Could you check a few things on this model? Use its own coordinates, in mm. Round coordinates to 2 decimals unless told otherwise and drop trailing zeros. Order: outer loops, then holes, each group sorted by start corner. A loop starts at its lowest first (then second) coordinate and runs counter-clockwise, first axis right, second up. Notation, with made-up numbers: (-15.5, 14) - (7.5, 14) arc R7 ccw to (7.5, 18) - close; hole circle Ø4 at (-1.5, 52.25). An arc over 180 degrees is marked (long way). Use one line per item in the form item = value.
from build123d import *

# Parameters (mm, degrees)
ESQUISSE1_W             = 366
ESQUISSE1_H             = 166
ESQUISSE1_R             = 2.2
ESQUISSE1_R_2           = 4.5
ESQUISSE1_R_3           = 6.5
BOSS_EXTRU_1_DEPTH      = 3
ESQUISSE2_OUTSIDE_W     = 448.38
ESQUISSE2_OUTSIDE_H     = 248.38
ESQUISSE2_OUTSIDE_W_2   = 222
ESQUISSE2_OUTSIDE_H_2   = 48
ENL_V_MAT_EXTRU_1_DEPTH = 4
CONG_1_R                = 6


with BuildPart() as part:
    # Esquisse1 → Boss.-Extru.1 (new body)
    with BuildSketch(Plane.XY):
        with Locations((183, 83)):
            Rectangle(ESQUISSE1_W, ESQUISSE1_H)
        with Locations((13, 153)):
            Circle(ESQUISSE1_R, mode=Mode.SUBTRACT)
        with Locations((13, 13)):
            Circle(ESQUISSE1_R, mode=Mode.SUBTRACT)
        with Locations((13, 83)):
            Circle(ESQUISSE1_R, mode=Mode.SUBTRACT)
        with Locations((173, 153)):
            Circle(ESQUISSE1_R, mode=Mode.SUBTRACT)
        with Locations((193, 83)):
            Circle(ESQUISSE1_R, mode=Mode.SUBTRACT)
        with Locations((173, 83)):
            Circle(ESQUISSE1_R, mode=Mode.SUBTRACT)
        with Locations((193, 153)):
            Circle(ESQUISSE1_R, mode=Mode.SUBTRACT)
        with Locations((353, 83)):
            Circle(ESQUISSE1_R, mode=Mode.SUBTRACT)
        with Locations((353, 13)):
            Circle(ESQUISSE1_R, mode=Mode.SUBTRACT)
        with Locations((353, 153)):
            Circle(ESQUISSE1_R, mode=Mode.SUBTRACT)
        with Locations((193, 13)):
            Circle(ESQUISSE1_R, mode=Mode.SUBTRACT)
        with Locations((173, 13)):
            Circle(ESQUISSE1_R, mode=Mode.SUBTRACT)
        with Locations((270.5, 83)):
            Circle(ESQUISSE1_R_2, mode=Mode.SUBTRACT)
        with Locations((95.5, 83)):
            Circle(ESQUISSE1_R_2, mode=Mode.SUBTRACT)
        with Locations((77.5, 101)):
            Circle(ESQUISSE1_R, mode=Mode.SUBTRACT)
        with Locations((113.5, 101)):
            Circle(ESQUISSE1_R, mode=Mode.SUBTRACT)
        with Locations((77.5, 65)):
            Circle(ESQUISSE1_R, mode=Mode.SUBTRACT)
        with Locations((113.5, 65)):
            Circle(ESQUISSE1_R, mode=Mode.SUBTRACT)
        with Locations((288.5, 65)):
            Circle(ESQUISSE1_R, mode=Mode.SUBTRACT)
        with Locations((252.5, 65)):
            Circle(ESQUISSE1_R, mode=Mode.SUBTRACT)
        with Locations((252.5, 101)):
            Circle(ESQUISSE1_R, mode=Mode.SUBTRACT)
        with Locations((288.5, 101)):
            Circle(ESQUISSE1_R, mode=Mode.SUBTRACT)
        with Locations((37, 49)):
            Circle(ESQUISSE1_R_3, mode=Mode.SUBTRACT)
        with Locations((61, 49)):
            Circle(ESQUISSE1_R_3, mode=Mode.SUBTRACT)
        with Locations((85, 49)):
            Circle(ESQUISSE1_R, mode=Mode.SUBTRACT)
        with Locations((13, 49)):
            Circle(ESQUISSE1_R, mode=Mode.SUBTRACT)
    extrude(amount=BOSS_EXTRU_1_DEPTH)

    # Esquisse2 outside → Enlèv. mat.-Extru.1 (cut, through all)
    with BuildSketch(Plane.XY.offset(3)):
        with Locations((183, 83)):
            Rectangle(ESQUISSE2_OUTSIDE_W, ESQUISSE2_OUTSIDE_H)
        with Locations((183, 83)):
            Rectangle(ESQUISSE2_OUTSIDE_W_2, ESQUISSE2_OUTSIDE_H_2, mode=Mode.SUBTRACT)
    extrude(amount=-ENL_V_MAT_EXTRU_1_DEPTH, mode=Mode.SUBTRACT)

    # Congé1
    cong_1_edges = [part.edges().sort_by_distance(p)[0] for p in [
        (72, 107, 1.5),
        (294, 107, 1.5),
        (294, 59, 1.5),
        (72, 59, 1.5),
    ]]
    fillet(cong_1_edges, radius=CONG_1_R)


solid = part.part
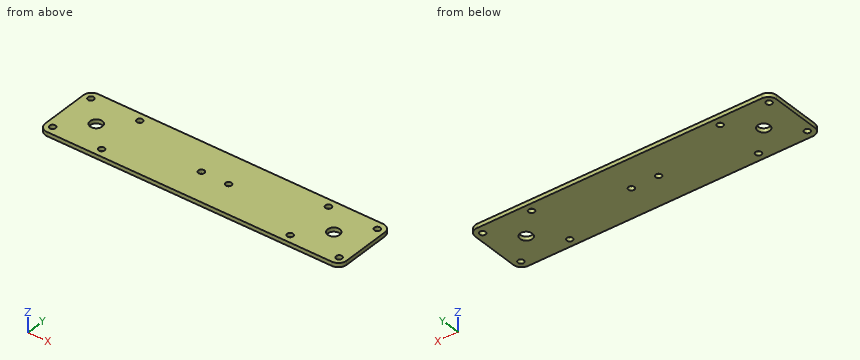
Item 1: I need wall thicknesses on L1, parallel to Y at x = 288.5, z = 0.75; L2, parallel to X at y = 81.5, z = 2.2; L3, parallel to X at y = 100, z = 0.65. Which ranges of each line are inside material? Lowest first, please.
Found:
L1 = 59.02 to 62.8, 67.2 to 98.8, 103.2 to 106.98
L2 = 72 to 91.26, 99.74 to 171.39, 174.61 to 191.39, 194.61 to 266.26, 274.74 to 294
L3 = 72 to 75.54, 79.46 to 111.54, 115.46 to 250.54, 254.46 to 286.54, 290.46 to 294
Item 2: Imagine slicing it at A-A on x = 113.5. Please give me the cut outline in (y, z).
Found:
outline = (59, 0) - (62.8, 0) - (62.8, 3) - (59, 3) - close; (67.2, 0) - (98.8, 0) - (98.8, 3) - (67.2, 3) - close; (103.2, 0) - (107, 0) - (107, 3) - (103.2, 3) - close
Item 3: Imagine slicing it at B-B on z = 2.1. State how many separate pieces and enclosed holes the cut face has, plus the area to 3 significant figures.
Found:
separate_pieces = 1
enclosed_holes = 12
area = 10,300 mm2
